Could you check a few things on this model? Use its own coordinates, in mm. Coordinates: 2 decimals unless noted, no trailing zeros. Order: outer loops, then holes, each group sorted by start corner. A loop starts at its lowest first (then second) coordinate and runs counter-clockwise, first axis right, second up. Notation, with made-up numbers: (-5, 38) -> (54, 38) arc R27 ccw to (54, 72) -> close; hole circle Ø8 at (23.25, 43). An arc over 180 degrees is marked (long way). Use a Markdown table: item, result. Add a question column.
1) If I drill on L1, parallel to Z at x = 0, y = -6.5; L2, parallel to Z at x = 21, y = 3; L3, parallel to X at y = -5, z = -10, over which ranges is the centre line in solid material (lowest first)? Write a range as [from, to].
2) If we section it at C-C (z = -27.5): Write out the boundary of the cut face in (x, y), plus the area to 3 significant figures.
3) If we section it at A-A (y = 0): Write out the boundary of the cut face in (x, z).
4) If we section it at D-D (z = -1.5): Write out the boundary of the cut face in (x, y).
5) Thinking about a two-plate mould opening in Z: for faces 1 (the cylindrical face through (-0.54, -2.44, 3.42)), 2 (the flat face through (-3, 0, 2.922)), 3 (the conical face through (2.961, -9.403, -13.024)), which applies, +Z half, -Z half, draft (parallel to the pull), parting line (faces both ways), or undercut?
6) Will these pins go through, and if not, where does the flat tip stop? pin 1 Ø10 at (x, z) = (9, -19.5) entering from -Y; pin 2 Ø10 at (y, z) = (6.5, -3) entering from +X; pin 3 Ø3 at (y, z) = (-3.5, -25) entering from +X.
```python
from build123d import *

# Parameters (mm, degrees)
F2_R     = 2.5
F3_DEPTH = 1


with BuildPart() as f1:
    # F0 (on Right) → F1 (revolve)
    with BuildSketch(Plane.YZ):
        with BuildLine():
            Line((0, 2.922098), (-13.120043, 2.922098))
            Line((-13.120043, 2.922098), (-7.84326, -22.875503))
            ThreePointArc((-7.84326, -22.875503), (-8.452987, -26.447656), (-11.315567, -28.669745))
            Line((-11.315567, -28.669745), (-26.197754, -33.098966))
            Line((-26.197754, -33.098966), (0, -33.098966))
            Line((0, -33.098966), (0, 2.922098))
        make_face()
    revolve(axis=Axis((0, 0, -15.088434), (0, 0, 1)))

    # F2 (on face) → F3 (join)
    with BuildSketch(Plane.XY.offset(2.922098)):
        Circle(F2_R)
    extrude(amount=F3_DEPTH)


solid = f1.part
```
Answer sheet:
| question | item | result |
|---|---|---|
| 1 | L1 | [-33.1, 2.92] |
| 1 | L2 | [-33.1, -31.62] |
| 1 | L3 | [-9.21, 9.21] |
| 2 | outline | circle Ø18.59 at (0, 0) |
| 2 | area | 271 mm2 |
| 3 | outline | (-26.2, -33.1) -> (26.2, -33.1) -> (11.32, -28.67) arc R5 cw to (7.84, -22.88) -> (13.12, 2.92) -> (2.5, 2.92) -> (2.5, 3.92) -> (-2.5, 3.92) -> (-2.5, 2.92) -> (-13.12, 2.92) -> (-7.84, -22.88) arc R5 cw to (-11.32, -28.67) -> close |
| 4 | outline | circle Ø24.43 at (0, 0) |
| 5 | face 1 | draft |
| 5 | face 2 | +Z half |
| 5 | face 3 | undercut |
| 6 | pin 1 | y = -7.78 |
| 6 | pin 2 | x = 12.28 |
| 6 | pin 3 | x = 7.9 |
